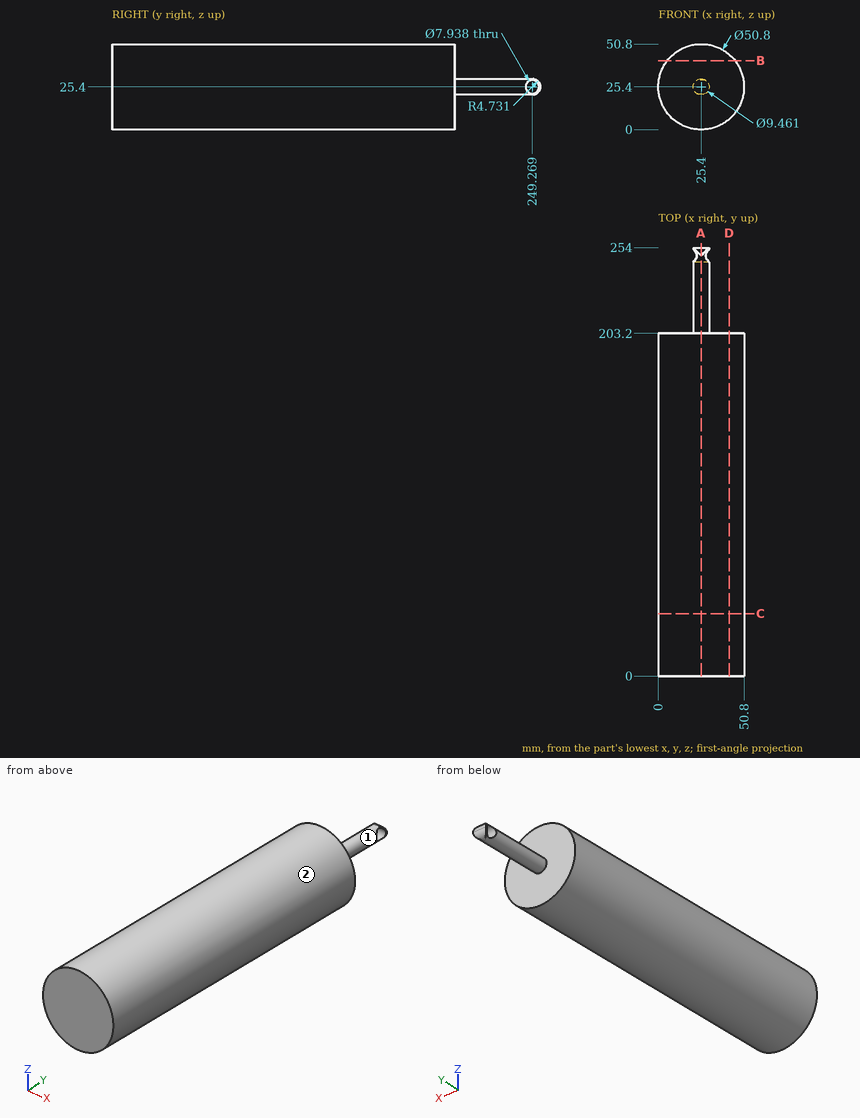
Input: dimensioned drawing with shaded views. Units: mm. Origin: part minimum x, y, z. A direction names the side the tool comes from. Coordinates: 2 decimals unless noted, no trailing zeros. Loops run counter-clockwise (first coordinate to the right, second up) from the corner with the lowest first, then second, coordinate; pieces in that order, holes last. Notation, with made-up numbers: (-21, 0.5) - (-12, 0.5) arc R5 ccw to (-12, 8.5) - close; hole circle Ø8 at (-7, 71). An arc over 180 degrees is marked (long way). One line per question, with ' | ' between items. Start each with the question number.
(1) Cut plane A-A on x = 25.4. Output: boundary loops of the cut face in (y, z), and give its area (3 significant figures).
(2) First-contact query: pin 1 (1 mm diameter, centred on x = 42, y = 147.5, fed in from +Z) (1 decimal); pin 2 (4 mm diameter, centred on y = 176.5, z = 29.5, fed in from -X); pin 3 (8 mm diameter, centred on y = 220, z = 22.5, fed in from +X). Flat tips, straight axial feed; report the tip coordinate or a pass-through.
(3) Ray query, L1, parallel to Y at x = 14.5, z = 16; L2, parallel to X at y = 117, z = 25.5; L3, parallel to Z at x = 24, y = 66.5. Return the intervals inside material, ascending. Write a range as from..to.
(4) Cut plane B-B on z = 41. Output: boundary loops of the cut face in (x, y) (1 decimal).
(5) Reachability of the marked faces 1 and 2 from +Z, -Z, +X, -X, +Y, -Y: full face, straight path, thin tool, end or side. Return the list, or none.
(6) Cut plane D-D on x = 42. Output: boundary loops of the cut face in (y, z) (1 decimal).
(7) Cut plane C-C on y = 37. Output: boundary loops of the cut face in (x, z), and give its area (3 significant figures).
Here are the results:
1) outline: (0, 0) - (203.2, 0) - (203.2, 20.67) - (249.27, 20.67) arc R4.73 ccw to (249.27, 30.13) - (203.2, 30.13) - (203.2, 50.8) - (0, 50.8) - close; hole circle Ø7.94 at (249.27, 25.4) | area: 10,700 mm²
2) pin 1: z = 45 | pin 2: x = 0.09 | pin 3: x = 30.13
3) L1: 0..203.2 | L2: 0..50.8 | L3: 0.04..50.76
4) outline: (5.4, 0) - (45.4, 0) - (45.4, 203.2) - (5.4, 203.2) - close
5) face 1: +Y | face 2: +Y, -Y
6) outline: (0, 6.2) - (203.2, 6.2) - (203.2, 44.6) - (0, 44.6) - close
7) outline: circle Ø50.8 at (25.4, 25.4) | area: 2,030 mm²
